from build123d import *

# Parameters (mm, degrees)
SKETCH1_W           = 20
SKETCH1_H           = 10
BOSS_EXTRUDE1_DEPTH = 30
SKETCH2_W           = 40
SKETCH2_H           = 40
BOSS_EXTRUDE2_DEPTH = 20
FILLET1_R           = 10


with BuildPart() as part:
    # Sketch1 → Boss-Extrude1 (new body)
    with BuildSketch(Plane.XY):
        with Locations((-20, -5)):
            Rectangle(SKETCH1_W, SKETCH1_H)
    extrude(amount=BOSS_EXTRUDE1_DEPTH)

    # Sketch2 → Boss-Extrude2 (add)
    with BuildSketch(Plane.XY):
        with Locations((-10, 10)):
            Rectangle(SKETCH2_W, SKETCH2_H)
    extrude(amount=-BOSS_EXTRUDE2_DEPTH)

    # Fillet1
    fillet1_edges = [part.edges().sort_by_distance(p)[0] for p in [
        (-20, 0, 0),
        (10, 30, -10),
        (-20, 0, 30),
    ]]
    fillet(fillet1_edges, radius=FILLET1_R - 0.0001)  # a hair under: the kernel refuses the full size


solid = part.part
Design review of the part built by this model. Coordinates are the model's own, in mm. A direction names the side the tool comes from. Give positions to 0.01 mm unless a question says otherwise; leave off trailing zeros. Loops run counter-clockwise (first coordinate to the right, second up) from the corner with the lowest first, then second, coordinate; pieces in that order, holes last. Notation, with made-up numbers: M -39.5,37.25 L -20.5,37.25 A23 cw -20.5,59.25 Z; hole C 7,-9 d8. An arc over 180 degrees is marked long. One line per question, with ' | ' between items. Start each with the question number.
1. To check wall thickness, follow L1, parallel to Y at x = -13, z = 15.5; L2, parallel to Z at x = 0, y = -4; L3, parallel to X at y = -8, z = 8.5. State the ranges of each line that lie inside material, in increasing order.
2. Add section D-D (y = 4). Write out the cut boundary in (x, z).
3. For faces 1 (the face through (7.15, 26.99, -10.14)), 2 (the face through (-20, 0, 15)), 3 (the face through (-6, 15, 0)), 4 (the face through (-10, -5, 15)), list the 3-axis set-ups (+Z, -Z, +X, -X, +Y, -Y) from which the entire face can be reached by the end or side of a thin tool; tool diameter is ignored.
4. Add section B-B (z = 12). Write out the cut boundary in (x, y), plus the area to 3 significant figures.
5. Add section C-C (y = 16.5). Write out the cut boundary in (x, z), plus the area to 3 significant figures.
6. Insertion check: P1, Ø8, axis at x = -16.5, z = 17, coming from the +Y side; P2, Ø10, axis at y = 4, z = 20, coming from the +X side; P3, Ø12, axis at x = -25.5, y = 21, coming from the +Z side. Each pin has a flat end and moves straight along its axis. Give the tip position at first contact, or say it passes through.
Worked out:
1) L1: y = -10 to 0 | L2: z = -20 to 0 | L3: x = -30 to -10
2) outline: M -30,-20 L 10,-20 L 10,0 L -10,0 L -10,2 L -30,2 Z
3) face 1: +Z, -Z, +X, +Y | face 2: +Z, +X, -X, +Y | face 3: +Z, +X, +Y | face 4: +Z, +X, +Y, -Y
4) outline: M -30,-10 L -10,-10 L -10,0 L -30,0 Z | area: 200 mm²
5) outline: M -30,-20 L 10,-20 L 10,0 L -30,0 Z | area: 800 mm²
6) P1: stops at y = 0 | P2: stops at x = -10 | P3: stops at z = 0
